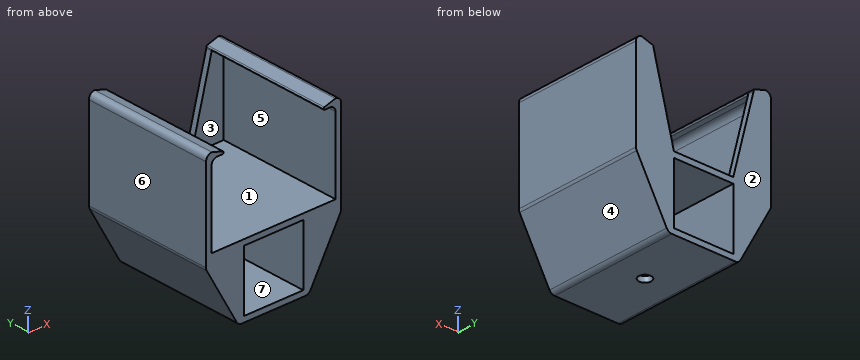
```python
from build123d import *

# Parameters (mm, degrees)
SALIENTE_EXTRUIR1_DEPTH             = 2
SALIENTE_EXTRUIR2_DEPTH             = 42
CORTAR_EXTRUIR1_REACH               = 46.1
CROQUIS3_W                          = 42
CROQUIS3_H                          = 27.1
CORTAR_EXTRUIR2_REACH               = 46.1
CROQUIS4_W                          = 27.1
CROQUIS4_H                          = 42
CROQUIS5_W                          = 20.2
CROQUIS5_H                          = 20.2
CORTAR_EXTRUIR3_DEPTH               = 45
DI_METRO_DE_TALADRO_4_2_4_2_1_D     = 4.2
DI_METRO_DE_TALADRO_4_2_4_2_1_DEPTH = 1.9
REDONDEO1_R                         = 0.4
REDONDEO2_R                         = 1.9
REDONDEO3_R                         = 2


with BuildPart() as part:
    # Croquis1 → Saliente-Extruir1 (new body)
    with BuildSketch(Plane(origin=(0, -115.999797701, 0), x_dir=(1, 0, 0), z_dir=(0, 1, 0))):
        with BuildLine():
            Line((10.1, -331), (17, -358.1))
            Line((17, -358.1), (17, -358.8))
            Line((17, -358.8), (21, -360))
            ThreePointArc((21, -360), (22.414213562, -359.414213562), (23, -358))
            Line((23, -358), (23, -327))
            Line((23, -327), (12, -307))
            Line((12, -307), (-12, -307))
            Line((-12, -307), (-23, -327))
            Line((-23, -327), (-23, -358))
            ThreePointArc((-23, -358), (-22.414213562, -359.414213562), (-21, -360))
            Line((-21, -360), (-17, -358.8))
            Line((-17, -358.8), (-17, -358.1))
            Line((-17, -358.1), (-10.1, -331))
            Line((-10.1, -331), (10.1, -331))
        make_face()
    extrude(amount=-SALIENTE_EXTRUIR1_DEPTH)

    # Croquis2 → Saliente-Extruir2 (add)
    with BuildSketch(Plane.XZ.offset(117.999797701)):
        with BuildLine():
            Line((-17, 331), (17, 331))
            Line((17, 331), (17, 358.8))
            Line((17, 358.8), (21, 360))
            ThreePointArc((21, 360), (22.414213562, 359.414213562), (23, 358))
            Line((23, 358), (23, 327))
            Line((23, 327), (12, 307))
            Line((12, 307), (-12, 307))
            Line((-12, 307), (-23, 327))
            Line((-23, 327), (-23, 358))
            ThreePointArc((-23, 358), (-22.414213562, 359.414213562), (-21, 360))
            Line((-21, 360), (-17, 358.8))
            Line((-17, 358.8), (-17, 331))
        make_face()
    extrude(amount=SALIENTE_EXTRUIR2_DEPTH)

    # Croquis3 → Cortar-Extruir1 (cut, up to next)
    with BuildSketch(Plane(origin=(-21.1, 0, 0), x_dir=(0, -1, 0), z_dir=(-1, 0, 0)), mode=Mode.PRIVATE) as cortar_extruir1_sk1:
        with Locations((138.999797701, 344.55)):
            Rectangle(CROQUIS3_W, CROQUIS3_H)
    cortar_extruir1_tool1 = extrude(cortar_extruir1_sk1.sketch, amount=-CORTAR_EXTRUIR1_REACH, mode=Mode.PRIVATE) & part.part
    add(cortar_extruir1_tool1.solids().sort_by_distance((-21.1, -138.999798, 344.55))[0], mode=Mode.SUBTRACT)

    # Croquis4 → Cortar-Extruir2 (cut, up to next)
    with BuildSketch(Plane(origin=(21.1, 0, 0), x_dir=(0, 0, -1), z_dir=(1, 0, 0)), mode=Mode.PRIVATE) as cortar_extruir2_sk1:
        with Locations((-344.55, -138.999797701)):
            Rectangle(CROQUIS4_W, CROQUIS4_H)
    cortar_extruir2_tool1 = extrude(cortar_extruir2_sk1.sketch, amount=-CORTAR_EXTRUIR2_REACH, mode=Mode.PRIVATE) & part.part
    add(cortar_extruir2_tool1.solids().sort_by_distance((21.1, -138.999798, 344.55))[0], mode=Mode.SUBTRACT)

    # Croquis5 → Cortar-Extruir3 (cut, through all)
    with BuildSketch(Plane(origin=(0, -115.999797701, 0), x_dir=(-1, 0, 0), z_dir=(0, 1, 0))):
        with Locations((0, 319)):
            Rectangle(CROQUIS5_W, CROQUIS5_H)
    extrude(amount=-CORTAR_EXTRUIR3_DEPTH, mode=Mode.SUBTRACT)

    # Diámetro de taladro Ø4.2 (4.2)1
    with Locations(Plane(origin=(0, 0, 307), x_dir=(-1, 0, 0), z_dir=(0, 0, -1))):
        with Locations((0, -137.999797701)):
            Hole(DI_METRO_DE_TALADRO_4_2_4_2_1_D / 2, depth=DI_METRO_DE_TALADRO_4_2_4_2_1_DEPTH)

    # Redondeo1
    redondeo1_edges = [part.edges().sort_by_distance(p)[0] for p in [
        (-17, -137.999797701, 358.8),
        (17, -137.999797701, 358.8),
        (-17, -138.999797701, 358.1),
        (17, -138.999797701, 358.1),
    ]]
    fillet(redondeo1_edges, radius=REDONDEO1_R)

    # Redondeo2
    redondeo2_edges = [part.edges().sort_by_distance(p)[0] for p in [
        (-21.1, -138.999797701, 358.1),
        (21.1, -138.999797701, 358.1),
    ]]
    fillet(redondeo2_edges, radius=REDONDEO2_R)

    # Redondeo3
    redondeo3_edges = [part.edges().sort_by_distance(p)[0] for p in [
        (-23, -137.999797701, 327),
        (-12, -137.999797701, 307),
        (12, -137.999797701, 307),
        (23, -137.999797701, 327),
    ]]
    fillet(redondeo3_edges, radius=REDONDEO3_R)


solid = part.part
```
Could you check a few things on this model? Use its own coordinates, in mm. Face numbers are marked on the shaded views. A direction names the side the tool comes from. Give positions to 0.01 mm unless a question says otherwise; leave off trailing zeros. Loops run counter-clockwise (first coordinate to the right, second up) from the corner with the lowest first, then second, coordinate; pieces in that order, holes last. Notation, with made-up numbers: (69.25, -40) - (92.25, -40) arc R36 ccw to (92.25, -5) - close; hole circle Ø10 at (-16.75, -32). An arc over 180 degrees is marked (long way). Answer in a Markdown table with one row per item. Add a question column.
Q1. Which directions (+Z, -Z, +X, -X, +Y, -Y) give clear straight access to the entire face, cutting with the end or side of a thin tool? Please do the marked faces 5, 6 and 7.
Q2. If we section it at D-D (x = 13.5): List the corners of the cut face in (y, z) for me.
Q3. Please list where these lines run through material, in increasing order: L1, parallel to X at y = -152.5, z = 355.5; L2, parallel to Y at x = 0, z = 307.45; L3, parallel to Z at x = -2, y = -157.5. Write a range as from..to.
Q4. We'd pull the mould along Z, two halves only. Please class the marked faces 1, 2, 3 and 4: +Z half, -Z half, draft (parallel to the pull), parting line (faces both ways), or undercut.
Q5. If we section it at A-A (z = 319): List the corners of the cut face in (x, y) for me.
Q6. For pin 1 (8 mm diameter, centred on x = -4, z = 322.5, fed in from +Y); pin 2 (5.5 mm diameter, centred on x = -15.5, z = 348.5, fed in from -Y); pin 3 (2.5 mm diameter, centred on x = 0, y = -138, fed in from +Z); pin 4 (0.5 mm diameter, centred on x = -18, y = -138, fed in from -Z), each with a flat end and sliding along its axis, tell me the tip position at first contact or that it passes through.
Q7. If we section it at B-B (x = 0): List the corners of the cut face in (y, z) for me.
The answers:
| question | item | result |
|---|---|---|
| 1 | face 5 | -Y |
| 1 | face 6 | +Z, -Z, -X, +Y, -Y |
| 1 | face 7 | +Y, -Y |
| 2 | outline | (-160, 309.73) - (-116, 309.73) - (-116, 344.35) - (-118, 344.35) - (-118, 331) - (-160, 331) - close |
| 3 | L1 | x = -23..-21.1, 21.1..23 |
| 3 | L2 | y = -160..-140.1, -135.9..-116 |
| 3 | L3 | z = 307..308.9, 329.1..331 |
| 4 | face 1 | undercut |
| 4 | face 2 | draft |
| 4 | face 3 | undercut |
| 4 | face 4 | -Z half |
| 5 | outline | (-18.6, -160) - (-10.1, -160) - (-10.1, -116) - (-18.6, -116) - close; (10.1, -160) - (18.6, -160) - (18.6, -116) - (10.1, -116) - close |
| 6 | pin 1 | passes through |
| 6 | pin 2 | stops at y = -118 |
| 6 | pin 3 | stops at z = 331 |
| 6 | pin 4 | stops at z = 317.45 |
| 7 | outline | (-160, 307) - (-140.1, 307) - (-140.1, 308.9) - (-160, 308.9) - close; (-160, 329.1) - (-116, 329.1) - (-116, 331) - (-160, 331) - close; (-135.9, 307) - (-116, 307) - (-116, 308.9) - (-135.9, 308.9) - close |
